```python
from build123d import *

# Parameters (mm, degrees)
SKETCH1_R           = 75
SKETCH1_R_2         = 37
SKETCH1_R_3         = 1.5
SKETCH1_W           = 3
SKETCH1_H           = 5
BOSS_EXTRUDE1_DEPTH = 2


with BuildPart() as part:
    # Sketch1 → Boss-Extrude1 (new body)
    with BuildSketch(Plane.XY):
        Circle(SKETCH1_R)
        Circle(SKETCH1_R_2, mode=Mode.SUBTRACT)
        with Locations((0, -43)):
            Circle(SKETCH1_R_3, mode=Mode.SUBTRACT)
        with Locations((-37.239092363, -21.5)):
            Circle(SKETCH1_R_3, mode=Mode.SUBTRACT)
        with Locations((-37.239092363, 21.5)):
            Circle(SKETCH1_R_3, mode=Mode.SUBTRACT)
        with Locations((0, 43)):
            Circle(SKETCH1_R_3, mode=Mode.SUBTRACT)
        with Locations((37.239092363, 21.5)):
            Circle(SKETCH1_R_3, mode=Mode.SUBTRACT)
        with Locations((37.239092363, -21.5)):
            Circle(SKETCH1_R_3, mode=Mode.SUBTRACT)
        with Locations((0, -60)):
            Circle(SKETCH1_R_3, mode=Mode.SUBTRACT)
        with Locations((54.378467222, 25.357095704)):
            Circle(SKETCH1_R_3, mode=Mode.SUBTRACT)
        with Locations((-54.378467222, 25.357095704)):
            Circle(SKETCH1_R_3, mode=Mode.SUBTRACT)
        with Locations((0, -52.5)):
            Rectangle(SKETCH1_W, SKETCH1_H, mode=Mode.SUBTRACT)
        with Locations((0, -67.5)):
            Rectangle(SKETCH1_W, SKETCH1_H, mode=Mode.SUBTRACT)
        Polygon((49.213000894, 24.603466076), (44.681461959, 22.490374768), (45.949316744, 19.771451406), (50.48085568, 21.884542715), align=None, mode=Mode.SUBTRACT)
        Polygon((58.276078765, 28.829648694), (62.8076177, 30.942740002), (64.075472485, 28.223816641), (59.54393355, 26.110725333), align=None, mode=Mode.SUBTRACT)
        Polygon((-58.276078765, 28.829648694), (-62.8076177, 30.942740002), (-64.075472485, 28.223816641), (-59.54393355, 26.110725333), align=None, mode=Mode.SUBTRACT)
        Polygon((-49.213000894, 24.603466076), (-44.681461959, 22.490374768), (-45.949316744, 19.771451406), (-50.48085568, 21.884542715), align=None, mode=Mode.SUBTRACT)
    extrude(amount=BOSS_EXTRUDE1_DEPTH)


solid = part.part
```
Geometry check sheet. Reference: the model listing, model coordinates, mm. Give positions to 0.01 mm unless a question says otherwise; leave off trailing zeros. Loops run counter-clockwise (first coordinate to the right, second up) from the corner with the lowest first, then second, coordinate; pieces in that order, holes last. Notation, with made-up numbers: M 0,-2 L 31,-2 A13 ccw 31,15 Z; hole C 27,45.25 d7. An arc over 180 degrees is marked long. Write item = value, one per line. Start each with the question number.
1. Thickness scan on probe 1 along X at (y, z) = (24.5, 1.1); probe 2 along Y at (x, z) = (-29.5, 0.8); probe 3 along X at (y, z) = (7.5, 1). Record the ranges inside material, lowest first.
2. Go/stop test with flat-tipped pins: P1, Ø4, axis at x = -37.24, y = -21.5, coming from the +Z side; P2, Ø1, axis at x = 0.5, z = 1, coming from the +Y side; P3, Ø1, axis at y = 45, z = 1.5, coming from the +X side; P4, Ø2.5, axis at x = -54.38, y = 25.36, coming from the +Z side. Record where each tip stops, or that it passes through.
3. Section check B-B, the plane x = -24. Enter the section's corners in (y, z), plus the area to 3 significant figures.
4. Draft check along Y on faces 1 (the face through (-8.02, -36.12, 0.99)), 2 (the face through (-9.764, 74.362, 0.986)), 3 (the face through (16, 34, 2)). Enter one of: +Y half, -Y half, draft (parallel to the pull), parting line (faces both ways), or undercut.
5. Section check A-A, the plane y = 0. Enter the section's corners in (x, z).
6. Section check C-C, the plane z = 1.7. Give the number of separate pieces and of enclosed holes in the cut face, plus the area to 3 significant figures.
Values follow:
q1.probe_1 = -70.89 to -55.61, -53.15 to -49.26, -48.99 to -27.73, 27.73 to 48.99, 49.26 to 53.15, 55.61 to 70.89
q1.probe_2 = -68.95 to -22.33, 22.33 to 68.95
q1.probe_3 = -74.62 to -36.23, 36.23 to 74.62
q2.P1 = 2
q2.P2 = 75
q2.P3 = 60.37
q2.P4 = through
q3.outline = M -71.06,0 L -28.16,0 L -28.16,2 L -71.06,2 Z; M 28.16,0 L 71.06,0 L 71.06,2 L 28.16,2 Z
q3.area = 172 mm^2
q4.face_1 = undercut
q4.face_2 = parting line
q4.face_3 = draft
q5.outline = M -75,0 L -37,0 L -37,2 L -75,2 Z; M 37,0 L 75,0 L 75,2 L 37,2 Z
q6.separate_pieces = 1
q6.enclosed_holes = 16
q6.area = 13,200 mm^2
